The listing builds one solid part. Answer for the finished solid, in the listing's coordinates (mm). A direction names the side the tool comes from. Coordinates: 2 decimals unless noted, no trailing zeros. Order: outer loops, then holes, each group sorted by start corner. A loop starts at its lowest first (then second) coordinate and runs counter-clockwise, first axis right, second up. Notation, with made-up numbers: (8.5, -12) -> (43.5, -12) arc R22 ccw to (43.5, -4) -> close; hole circle Ø1 at (20, 73.5). An arc over 180 degrees is marked (long way). Return JSON: item names as keys, results as strings.
```python
from build123d import *

# Parameters (mm, degrees)
F0_R     = 15.875
F1_DEPTH = 21
F2_R     = 1


# Not quite as in the source:
# - a feature names something its author has since deleted; it is built from what else it names


with BuildPart() as f1:
    # F0 (on Top) → F1 (new body)
    with BuildSketch(Plane.XY):
        Circle(F0_R)
        with BuildLine():
            ThreePointArc((6.1426785688, 13.3), (12.3412467165, 7.8940565924), (14.65, 0))
            ThreePointArc((14.65, 0), (-7.8940565924, -12.3412467165), (-6.1426785688, 13.3))
            ThreePointArc((-6.1426785688, 13.3), (0, 14.65), (6.1426785688, 13.3))
        make_face(mode=Mode.SUBTRACT)
        with BuildLine():
            Line((-6.1426785688, 13.3), (6.1426785688, 13.3))
            ThreePointArc((6.1426785688, 13.3), (0, 14.65), (-6.1426785688, 13.3))
        make_face()
    extrude(amount=F1_DEPTH)

    # F2
    f2_edges = [f1.edges().sort_by_distance(p)[0] for p in [
        (0, -14.65, 21),
        (0, 13.3, 21),
        (0, -14.65, 0),
        (0, 13.3, 0),
    ]]
    fillet(f2_edges, radius=F2_R)


solid = f1.part
```
Item 1: Which of the six approach directions +Z, -Z, +X, -X, +Y, -Y give full straight-line access (tool end or side, diameter ignored) to faces 4 (the flat face through (1, 15, 21)), 5 (the flat face through (0, 13.3, 10)), 6 (the cylindrical face through (0.089, 13.585, 0.301))?
Answer list:
{"face 4": "+Z, +X, -X, +Y, -Y", "face 5": "+Z, -Z", "face 6": "-Z"}
Item 2: The part is cut by section A-A on z = 12. Determine the outline of the cut face in (x, y) (3 decimals).
Answer list:
{"outline": "circle Ø31.75 at (0, 0); hole (-6.143, 13.3) arc R14.65 ccw (long way) to (6.143, 13.3) -> close"}
Item 3: Find the intervals of material crossed by probe 1 along Y at (x, z) = (0, 16) (3 decimals); probe 2 along Y at (x, z) = (-11, 11); probe 3 along X at (y, z) = (-3, 6.25), in increasing order.
Answer list:
{"probe 1": "-15.875 to -14.65, 13.3 to 15.875", "probe 2": "-11.45 to -9.68, 9.68 to 11.45", "probe 3": "-15.59 to -14.34, 14.34 to 15.59"}
Item 4: Determine the mould class of faces 1 (the cylindrical face through (0.089, 13.585, 20.699)), 2 (the flat face through (1, 15, 0)), 3 (the cylindrical face through (-3.441, -15.497, 10.353)) for opening direction Y: pulls with the +Y half, pulls with the -Y half, needs draft (parallel to the pull), parting line crosses it, or undercut.
Answer list:
{"face 1": "undercut", "face 2": "needs draft", "face 3": "parting line crosses it"}
Item 5: Flat-ended cylindrical pins translate along their axes: pin 1 (3 mm diameter, centred on x = -12, z = 13.5, fed in from +Y); pin 2 (3.5 mm diameter, centred on x = -2.5, z = 11, fed in from -Y); pin 3 (5 mm diameter, centred on x = -9.5, y = -8.5, fed in from -Z); pin 4 (12 mm diameter, centred on x = -4, y = 11.5, fed in from -Z). Find the tip coordinate at first contact, or state that the pin passes through.
Answer list:
{"pin 1": "y = 11.91", "pin 2": "y = -15.86", "pin 3": "z = 0.08", "pin 4": "z = 0"}
